Geometry: final body of the model. Coordinates: model frame, mm. Face numbers are marked on the shaded views. A direction names the side the tool comes from. Give positions to 0.01 mm unless a question says otherwise; leave off trailing zeros. Loops run counter-clockwise (first coordinate to the right, second up) from the corner with the lowest first, then second, coordinate; pieces in that order, holes last. Notation, with made-up numbers: (24, -11.75) - (51, -11.75) arc R10 ccw to (51, 3.25) - close; hole circle Ø11 at (-25, -38). An arc over 180 degrees is marked (long way). Use one line per item in the form item = value.
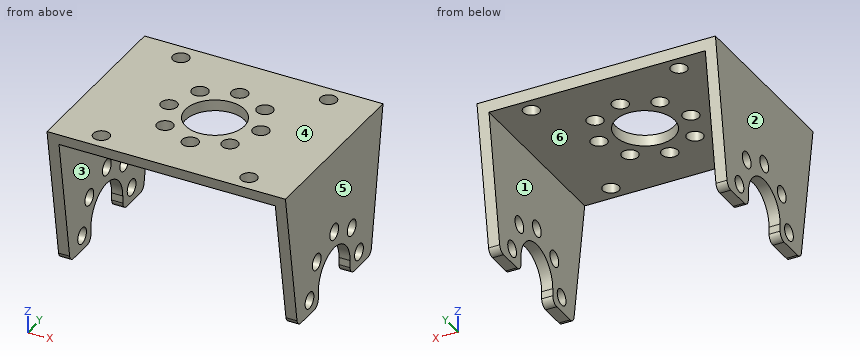
```python
from build123d import *

# Parameters (mm, degrees)
F1_DEPTH = 25
F2_R     = 1.1
F3_DEPTH = 32.301
F4_R     = 1.1
F4_R_2   = 4
F5_DEPTH = 1.5
F6_R     = 1


with BuildPart() as f1:
    # F0 (on Front) → F1 (new body)
    with BuildSketch(Plane.XZ):
        Polygon((0, 19.5), (0, 0), (1.5, 0), (1.5, 18), (30.8, 18), (30.8, 0), (32.3, 0), (32.3, 19.5), align=None)
    extrude(amount=F1_DEPTH)

    # F2 (on face) → F3 (cut, through all)
    with BuildSketch(Plane(origin=(0, 0, 0), x_dir=(0, -1, 0), z_dir=(-1, 0, 0))):
        with BuildLine():
            Line((16.5, 0), (16.5, 2))
            ThreePointArc((16.5, 2), (12.5, 6), (8.5, 2))
            Line((8.5, 2), (8.5, 0))
            Line((8.5, 0), (16.5, 0))
        make_face()
        with Locations((18.7225396744, 2)):
            Circle(F2_R)
        with Locations((16.9, 6.4)):
            Circle(F2_R)
        with Locations((12.5, 8.2225396744)):
            Circle(F2_R)
        with Locations((8.1, 6.4)):
            Circle(F2_R)
        with Locations((6.2774603256, 2)):
            Circle(F2_R)
        Polygon((0, 0), (3.2774603256, 0), (0, 21), align=None)
        Polygon((21.7225396744, 0), (25, 0), (25, 21), align=None)
    extrude(amount=-F3_DEPTH, mode=Mode.SUBTRACT)

    # F4 (on face) → F5 (cut, through all)
    with BuildSketch(Plane.XY.offset(19.5)):
        with Locations((6.15, -2.5)):
            Circle(F4_R)
        with Locations((26.15, -2.5)):
            Circle(F4_R)
        with Locations((6.15, -22.5)):
            Circle(F4_R)
        with Locations((26.15, -22.5)):
            Circle(F4_R)
        with Locations((16.15, -12.5)):
            Circle(F4_R_2)
        with Locations((11.75, -8.1)):
            Circle(F4_R)
        with Locations((9.9274603256, -12.5)):
            Circle(F4_R)
        with Locations((11.75, -16.9)):
            Circle(F4_R)
        with Locations((16.15, -18.7225396744)):
            Circle(F4_R)
        with Locations((20.55, -16.9)):
            Circle(F4_R)
        with Locations((22.3725396744, -12.5)):
            Circle(F4_R)
        with Locations((20.55, -8.1)):
            Circle(F4_R)
        with Locations((16.15, -6.2774603256)):
            Circle(F4_R)
    extrude(amount=-F5_DEPTH, mode=Mode.SUBTRACT)

    # F6
    f6_edges = [f1.edges().sort_by_distance(p)[0] for p in [
        (31.55, -3.27746, 0),
        (0.75, -3.27746, 0),
        (0.75, -8.5, 0),
        (31.55, -8.5, 0),
        (0.75, -16.5, 0),
        (31.55, -16.5, 0),
        (0.75, -21.72254, 0),
        (31.55, -21.72254, 0),
    ]]
    fillet(f6_edges, radius=F6_R)


solid = f1.part
```
(1) Cut plane D-D (x = 16.15). Return the cut outline in (y, z).
Solution:
outline = (-24.77, 19.5) - (-24.53, 18) - (-19.82, 18) - (-19.82, 19.5) - close; (-17.62, 18) - (-16.5, 18) - (-16.5, 19.5) - (-17.62, 19.5) - close; (-8.5, 18) - (-7.38, 18) - (-7.38, 19.5) - (-8.5, 19.5) - close; (-5.18, 18) - (-0.47, 18) - (-0.23, 19.5) - (-5.18, 19.5) - close
(2) Cut plane B-B (y = -12.5). Return the cut outline in (x, z).
Solution:
outline = (0, 6) - (1.5, 6) - (1.5, 7.12) - (0, 7.12) - close; (0, 9.32) - (1.5, 9.32) - (1.5, 18) - (8.83, 18) - (8.83, 19.5) - (0, 19.5) - close; (11.03, 18) - (12.15, 18) - (12.15, 19.5) - (11.03, 19.5) - close; (20.15, 18) - (21.27, 18) - (21.27, 19.5) - (20.15, 19.5) - close; (23.47, 18) - (30.8, 18) - (30.8, 9.32) - (32.3, 9.32) - (32.3, 19.5) - (23.47, 19.5) - close; (30.8, 6) - (32.3, 6) - (32.3, 7.12) - (30.8, 7.12) - close
(3) Pin query (flat end, axial travel): P1, Ø3, axis at x = 20.55, y = -8.1, coming from the -Z side; P2, Ø2, axis at x = 16.15, y = -18.72, coming from the +Z side; P3, Ø4, axis at x = 16.5, z = 16.5, coming from the -Y side; P4, Ø0.5, axis at x = 31.5, z = 1.5, coming from the +Y side. Return the tip coordinate at first contact, or that it passes through.
Solution:
P1 = 18
P2 = through
P3 = -24.61
P4 = -3
(4) Pull-direction query (X, two-part tool) for the marked faces 1, 2, 3 and 4; classes: released by +X, released by -X, zero draft, split by the parting line, or undercut.
Solution:
face_1 = undercut
face_2 = released by -X
face_3 = undercut
face_4 = zero draft
(5) Cut plane A-A (x = 6.15). Return the cut outline in (y, z).
Solution:
outline = (-24.77, 19.5) - (-24.53, 18) - (-23.6, 18) - (-23.6, 19.5) - close; (-21.4, 18) - (-3.6, 18) - (-3.6, 19.5) - (-21.4, 19.5) - close; (-1.4, 18) - (-0.47, 18) - (-0.23, 19.5) - (-1.4, 19.5) - close
(6) Cut plane C-C (y = -8.1). Return the cut outline in (x, z).
Solution:
outline = (0, 0.2) - (1.5, 0.2) - (1.5, 5.3) - (0, 5.3) - close; (0, 7.5) - (1.5, 7.5) - (1.5, 18) - (10.65, 18) - (10.65, 19.5) - (0, 19.5) - close; (12.85, 18) - (19.45, 18) - (19.45, 19.5) - (12.85, 19.5) - close; (21.65, 18) - (30.8, 18) - (30.8, 7.5) - (32.3, 7.5) - (32.3, 19.5) - (21.65, 19.5) - close; (30.8, 0.2) - (32.3, 0.2) - (32.3, 5.3) - (30.8, 5.3) - close
(7) Material intervals for L1, parallel to X at y = -2.5, z = 8.5; L2, parallel to Y at x = 16.15, z = 18.75; L3, parallel to Y at x = 6.15, z = 19.15, sorted ascending. Write a range as from..to.
Solution:
L1 = 0..1.5, 30.8..32.3
L2 = -24.65..-19.82, -17.62..-16.5, -8.5..-7.38, -5.18..-0.35
L3 = -24.71..-23.6, -21.4..-3.6, -1.4..-0.29
(8) Access query for the marked faces 5 and 6. Directions: +Z, -Z, +X, -X, +Y, -Y. A direction counts if a zero-diameter tool reaches every point of the face in a straight line with its end or side. Return the directions, or none.
Solution:
face_5 = +Z, -Z, +X, +Y, -Y
face_6 = -Z, +Y, -Y
